For this review, take the finished solid that the model builds, in its own axes (mm). Coordinates: 2 decimals unless noted, no trailing zeros. Write each loop counter-clockwise with the first axis right and the second up, starting at its lowest first coordinate (ties: lowest second). Pieces come first, ordered by that corner, then holes.
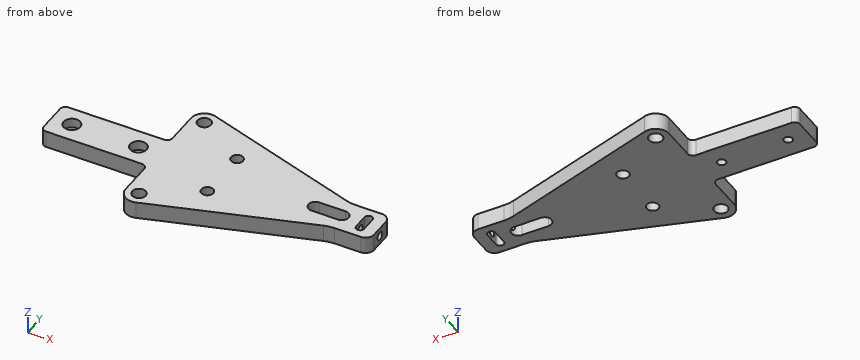
Autodesk Inventor part; units mm, degrees
ref_plane "YZ Plane" through (0, 0, 0) normal (1, 0, 0) x (0, 1, 0)
ref_plane "XY Plane" through (0, 0, 0) normal (0, 0, 1) x (1, 0, 0)
sketch "Sketch1" plane through (0, 0, 0) normal (0, 0, 1) x (1, 0, 0)
  line L0 (-20, 150) -> (20, 150) construction
  line L1 (20, 150) -> (20, -150) construction
  line L2 (20, -150) -> (-20, -150) construction
  line L3 (-20, -150) -> (-20, 150) construction
  circle A0 centre (-30.5, 22) radius 11.95 construction
  circle A1 centre (-30.5, -22) radius 11.95 construction
  circle A2 centre (30.5, 0) radius 11.95 construction
  line L4 (42.45, 4.056) -> (42.45, -13.1126) construction
  circle A3 centre (30.5, 0) radius 7.5
  circle A4 centre (-30.5, 22) radius 5
  circle A5 centre (-30.5, -22) radius 5
  line L5 (-35.5, 3.8118) -> (-35.5, -3.8118) construction
  line L6 (0, 150) -> (0, -150) construction
  line L7 (-20, -108) -> (-20, -150) construction
  line L8 (-20, 150) -> (-20, 108) construction
  line L9 (-75.5, 7.5) -> (-35.5, 7.5)
  line L10 (-35.5, 7.5) -> (-35.5, -7.5)
  line L11 (-35.5, -7.5) -> (-75.5, -7.5)
  line L12 (-75.5, -7.5) -> (-75.5, 7.5)
  circle A6 centre (0, -150) radius 6 construction
  circle A7 centre (-11.5, -10) radius 4.5
  circle A8 centre (0, -150) radius 7
  line L13 (-7, -150) -> (-7, -10)
  line L14 (-11.5, 5.5) -> (-180, 5.5)
  line L15 (-11.5, -5.5) -> (-180, -5.5)
  line L16 (-185.5, -10) -> (-35.5, -10) construction
  line L17 (-35.5, -10) -> (-35.5, 10) construction
  line L18 (-35.5, 10) -> (-185.5, 10) construction
  line L19 (-185.5, 10) -> (-185.5, -10) construction
  circle A9 centre (-180, 0) radius 4.5 construction
  circle A10 centre (-180, 0) radius 5.5
  circle A11 centre (-11.5, -10) radius 2.5 construction
  line L20 (-35.5, -22) -> (-35.5, 22)
  line L21 (-28.9863, -26.7654) -> (32.7706, -7.148)
  line L22 (-28.9863, 26.7654) -> (32.7706, 7.148)
  line L23 (-20, 0) -> (0, 0)
  circle A12 centre (0, 150) radius 4.5 construction
  circle A13 centre (0, 150) radius 7
  line L24 (-7, 150) -> (-7, 10)
  circle A14 centre (-11.5, 10) radius 4.5
  line L25 (7, -150) -> (7, 150)
  point P0 (20, 0)
  point P1 (-29.8, 0)
  point P2 (-35.4948, -21.7719)
  point P3 (-35.4948, 21.7719)
  point P4 (-28.5008, 26.5829)
  point P5 (32.6594, 7.1824)
  point P6 (32.6594, -7.1824)
  point P7 (-28.5008, -26.5829)
  point P8 (-35.5, 0)
  point P9 (-68, 0)
  point P10 (-43, 0)
  point P11 (-75.5, 0)
  point P12 (-35.5, 0)
  point P13 (-95.75, -5.5)
  point P14 (-185.5, 0)
  dimension "d0" = 40
  dimension "d1" = 300
  dimension "d2" = 23.9
  dimension "d3" = 22
  dimension "d4" = 22
  dimension "d6" = 30.5
  dimension "d7" = 30.5
  dimension "d12" = 15
  dimension "d38" = 10
  dimension "d42" = 15
  dimension "d43" = 40
  dimension "d44" = 25
  dimension "d45" = 7.5
  dimension "d46" = 7.5
  dimension "d48" = 12
  dimension "d49" = 9
  dimension "d51" = 1
  dimension "d53" = 20
  dimension "d55" = 9
  dimension "d56" = 1
  dimension "d60" = 150
  dimension "d74" = 9
  dimension "d75" = 2.5
  dimension "d76" = 9
extrude "Extrusion1" add sketch "Sketch1" against normal blind 6.35 contours A3 | A3 L21 L25 L22 | L25 L21 L13 A7 L15 L10 L14 A14 L24 L22 | L24 A14 L14 L10 L20 A4 L22 | L21 A5 L20 L10 L15 A7 L13 | A4 | A14 | A7 | A5 | L10 L14 L12 L9 | L10 L15 L12 L14 | L10 L11 L12 L15
hole "Hole1" at (-30.5, 22, 0) at (-30.5, -22, 0) at (30.5, 0, 0) direction (0, 0, -1) diameter 5.1 end through all
hole "Hole2" at (-43, 0, 0) at (-68, 0, 0) direction (0, 0, -1) diameter 3.2 end through all counterbore diameter 6.2 counterbore depth 3.58
fillet "Fillet1" radius 2 4 edges at (-75.5, 7.5, -3.175) (-75.5, -7.5, -3.175) (-35.5, -7.5, -3.175) (-35.5, 7.5, -3.175)
hole "Hole4" at (-11.5, -10, 0) at (-11.5, 10, 0) direction (0, 0, -1) diameter 4.5 end through all
sketch "Sketch3" plane through (0, 0, 0) normal (0, 0, 1) x (1, 0, 0)
  circle A0 centre (-11.5, -10) radius 2.25
  circle A1 centre (-11.5, 10) radius 2.25
  circle A2 centre (-43, 0) radius 3.1
  circle A3 centre (-68, 0) radius 3.1
  circle A4 centre (-30.5, 22) radius 2.55
  circle A5 centre (-30.5, -22) radius 2.55
  arc A6 (-75.5, -5.5) -> (-73.5, -7.5) centre (-73.5, -5.5) ccw
  line L0 (-73.5, -7.5) -> (-37.5, -7.5)
  arc A7 (-35.5, -9.5) -> (-37.5, -7.5) centre (-37.5, -9.5) ccw
  line L1 (-35.5, -9.5) -> (-35.5, -22)
  arc A8 (-35.5, -22) -> (-28.9863, -26.7654) centre (-30.5, -22) ccw
  line L2 (-28.9863, -26.7654) -> (32.7706, -7.148)
  arc A9 (32.7706, -7.148) -> (32.7706, 7.148) centre (30.5, 0) ccw
  line L3 (32.7706, 7.148) -> (-28.9863, 26.7654)
  arc A10 (-28.9863, 26.7654) -> (-35.5, 22) centre (-30.5, 22) ccw
  line L4 (-35.5, 22) -> (-35.5, 9.5)
  arc A11 (-37.5, 7.5) -> (-35.5, 9.5) centre (-37.5, 9.5) ccw
  line L5 (-37.5, 7.5) -> (-73.5, 7.5)
  arc A12 (-73.5, 7.5) -> (-75.5, 5.5) centre (-73.5, 5.5) ccw
  line L6 (-75.5, 5.5) -> (-75.5, -5.5)
  point P0 (0, 0)
sketch "Sketch4" plane through (0, 0, 0) normal (0, 0, 1) x (1, 0, 0)
  circle A0 centre (33.5, 0) radius 2.55 construction
  line L0 (33.5, 0) -> (23.5, 0) construction
  line L1 (33.5, 2.55) -> (23.5, 2.55)
  line L2 (23.5, -2.55) -> (33.5, -2.55)
  arc A1 (33.5, -2.55) -> (33.5, 2.55) centre (33.5, 0) ccw
  arc A2 (23.5, 2.55) -> (23.5, -2.55) centre (23.5, 0) ccw
  circle A3 centre (30.5, 0) radius 2.55
  point P0 (0, 0)
  point P1 (28.5, 0)
  point P2 (33.5, 2.55)
  dimension "d78" = 10
  dimension "d97" = 3
extrude "Extrusion2" cut sketch "Sketch4" against normal blind 25.4
sketch "Sketch5" plane through (0, 0, 0) normal (0, 0, 1) x (1, 0, 0)
  line L0 (32.7706, 7.148) -> (-28.9863, 26.7654)
  line L1 (32.7706, 7.148) -> (47.7706, 7.148)
  line L2 (47.7706, 7.148) -> (47.7706, -7.148)
  line L3 (47.7706, -7.148) -> (32.7706, -7.148)
  line L4 (-28.9863, -26.7654) -> (32.7706, -7.148)
  line L5 (40.4103, 2.8) -> (43.4103, 2.8)
  line L6 (43.4103, 2.8) -> (43.4103, -2.8)
  line L7 (43.4103, -2.8) -> (40.4103, -2.8)
  line L8 (40.4103, -2.8) -> (40.4103, 2.8)
  line L9 (36.05, 2.2796) -> (36.05, -2.3678) construction
  arc A0 (32.7706, -7.148) -> (32.7706, 7.148) centre (30.5, 0) ccw
  circle A1 centre (41.9103, 2.8) radius 1.5
  circle A2 centre (41.9103, -2.8) radius 1.5
  arc A3 (33.5, -2.55) -> (33.5, 2.55) centre (33.5, 0) ccw
  point P0 (0, 0)
  point P1 (32.7098, 0)
  point P2 (40.4103, 0)
  point P3 (43.4103, 2.8)
  point P4 (40.4103, 2.8)
  dimension "d81" = 3
  dimension "d82" = 5.6
  dimension "d83" = 15
  dimension "d84" = 4.3603
  dimension "d85" = 4.3603
extrude "Extrusion3" add sketch "Sketch5" against normal up to surface (6.35 mm away)
sketch "Sketch6" plane through (47.7706, -7.148, 0) normal (1, 0, 0) x (0, 0, -1)
  line L0 (6.35, 14.2961) -> (6.35, 0)
  line L1 (0, 14.2961) -> (6.35, 14.2961)
  line L2 (0, 0) -> (0, 14.2961)
  line L3 (0, 0) -> (6.35, 0)
  point P0 (0, 7.148)
  point P1 (3.175, 7.148)
  point P2 (0, 7.148)
  point P3 (3.175, 14.2961)
hole "Hole5" at (47.7706, 0, -3.175) direction (-1, 0, 0) diameter 3.2 depth 25.4 tip angle 118
fillet "Fillet2" radius 12.7 2 edges at (32.7706, 7.148, -3.175) (32.7706, -7.148, -3.175)
fillet "Fillet3" radius 3.175 2 edges at (47.7706, -7.148, -3.175) (47.7706, 7.148, -3.175)
sketch "Sketch7" plane through (0, 0, -6.35) normal (0, 0, -1) x (-1, 0, 0)
  arc A0 (-43.4103, -2.8) -> (-40.4103, -2.8) centre (-41.9103, -2.8) ccw
  line L0 (-43.4103, -2.8) -> (-43.4103, 2.8)
  arc A1 (-40.4103, 2.8) -> (-43.4103, 2.8) centre (-41.9103, 2.8) ccw
  line L1 (-40.4103, 2.8) -> (-40.4103, -2.8)
  line L2 (-33.5, 2.55) -> (-23.5, 2.55)
  arc A2 (-23.5, -2.55) -> (-23.5, 2.55) centre (-23.5, 0) ccw
  line L3 (-23.5, -2.55) -> (-33.5, -2.55)
  circle A3 centre (30.5, 22) radius 2.55
  circle A4 centre (30.5, -22) radius 2.55
  circle A5 centre (68, 0) radius 1.6
  circle A6 centre (43, 0) radius 1.6
  arc A7 (-44.5956, 7.148) -> (-47.7706, 3.973) centre (-44.5956, 3.973) ccw
  line L4 (-47.7706, 3.973) -> (-47.7706, -3.973)
  arc A8 (-47.7706, -3.973) -> (-44.5956, -7.148) centre (-44.5956, -3.973) ccw
  line L5 (-44.5956, -7.148) -> (-34.7392, -7.148)
  arc A9 (-30.8944, -7.744) -> (-34.7392, -7.148) centre (-34.7392, -19.848) ccw
  line L6 (-30.8944, -7.744) -> (28.9863, -26.7654)
  arc A10 (28.9863, -26.7654) -> (35.5, -22) centre (30.5, -22) ccw
  line L7 (35.5, -22) -> (35.5, -9.5)
  arc A11 (37.5, -7.5) -> (35.5, -9.5) centre (37.5, -9.5) ccw
  line L8 (37.5, -7.5) -> (73.5, -7.5)
  arc A12 (73.5, -7.5) -> (75.5, -5.5) centre (73.5, -5.5) ccw
  line L9 (75.5, -5.5) -> (75.5, 5.5)
  arc A13 (75.5, 5.5) -> (73.5, 7.5) centre (73.5, 5.5) ccw
  line L10 (73.5, 7.5) -> (37.5, 7.5)
  arc A14 (35.5, 9.5) -> (37.5, 7.5) centre (37.5, 9.5) ccw
  line L11 (35.5, 9.5) -> (35.5, 22)
  arc A15 (35.5, 22) -> (28.9863, 26.7654) centre (30.5, 22) ccw
  line L12 (28.9863, 26.7654) -> (-30.8944, 7.744)
  arc A16 (-34.7392, 7.148) -> (-30.8944, 7.744) centre (-34.7392, 19.848) ccw
  line L13 (-34.7392, 7.148) -> (-44.5956, 7.148)
  circle A17 centre (11.5, 10) radius 2.25
  circle A18 centre (11.5, -10) radius 2.25
  arc A19 (-33.5, 2.55) -> (-33.5, -2.55) centre (-33.5, 0) ccw
  point P0 (0, 0)
equation "\"d4\" = d3"
equation "\"d7\" = d6"
equation "\"CAM_OFFSET\" = -0.508"
properties part number "XZ Plate"
1) Consider section B-B (x = -30.5). Give the boundary of the cut face in (y, z).
2) Consider section C-C (y = 0). Count the separate pieces of the cut face and the enclosed holes in it, then the cut area to 3 significant figures.
3) For L1, parallel to X at y = 0, z = -2.5; L2, parallel to Y at x = -68, z = -1; L3, parallel to Y at x = -68, z = -5, list the stretches that pass through material, from the lowest coordinate up.
4) Consider section A-A (x = -43). Give the boundary of the cut face in (y, z).
5) Clearance check with flat-ended pins moving along their axes: P1, Ø8, axis at x = -68, y = 0, coming from the -Z side; P2, Ø1.9, axis at x = 27, z = -2.5, coming from the -Y side; P3, Ø4, axis at x = -11.5, y = -10, coming from the +Z side; P4, Ø1.9, axis at x = -42, y = 1, coming from the +Z side. State where each tip first meets the part, or that it passes through.
6) Consider section D-D (y = -15.5). Give the boundary of the cut face in (x, z).
Results:
1. outline: (-27, -6.35) - (-24.55, -6.35) - (-24.55, 0) - (-27, 0) - close; (-19.45, -6.35) - (19.45, -6.35) - (19.45, 0) - (-19.45, 0) - close; (24.55, -6.35) - (27, -6.35) - (27, 0) - (24.55, 0) - close
2. separate pieces: 7
2. enclosed holes: 0
2. area: 578 mm2
3. L1: x = -75.5 to -71.1, -64.9 to -46.1, -39.9 to 20.95
3. L2: y = -7.5 to -3.1, 3.1 to 7.5
3. L3: y = -7.5 to -1.6, 1.6 to 7.5
4. outline: (-7.5, -6.35) - (-1.6, -6.35) - (-1.6, -3.58) - (-3.1, -3.58) - (-3.1, 0) - (-7.5, 0) - close; (1.6, -6.35) - (7.5, -6.35) - (7.5, 0) - (3.1, 0) - (3.1, -3.58) - (1.6, -3.58) - close
5. P1: stops at z = -6.35
5. P2: stops at y = -9.28
5. P3: passes through
5. P4: stops at z = -3.58
6. outline: (-35.5, -6.35) - (6.48, -6.35) - (6.48, 0) - (-35.5, 0) - close
